The model under review builds one solid part; all positions refer to its coordinate system, in mm. A direction names the side the tool comes from. Coordinates: 2 decimals unless noted, no trailing zeros. Loops run counter-clockwise (first coordinate to the right, second up) from the corner with the lowest first, then second, coordinate; pieces in that order, holes last. Notation, with made-up numbers: M -19,17 L 15,17 A31 ccw 15,56 Z; hole C 35.5,39.5 d5. An arc over 180 degrees is marked long. Write item = value, one per line. Start each with the question number.
Q1. For faces 5 (the face through (12, 7, 3)), 6 (the face through (-7, 8, 2)), 7 (the face through (19, 8, 2)), 8 (the face through (10.566, 5.986, 1.394)), 9 (the face through (11, 7, 1)), list the 3-axis set-ups (+Z, -Z, +X, -X, +Y, -Y) from which the entire face can be reached by the end or side of a thin tool; tool diameter is ignored.
Q2. We need section A-A on y = 7.5. Give the boundary of the cut face in (x, z), and give its area (3 significant figures).
Q3. We need section D-D on y = 13.25. Give the boundary of the cut face in (x, z).
Q4. Wall thickness on probe 1 along Z at (x, y) = (4.5, 3.25); probe 2 along Y at (x, z) = (22, -1.4); probe 3 along X at (y, z) = (3.25, 2.75): over which ranges is each line inside the solid? List them lowest first.
Q5. We need section B-B on z = -1.5. Give the boundary of the cut face in (x, y), and give its area (3 significant figures).
Q6. We need section C-C on x = 26.5. Give the boundary of the cut face in (y, z), and give its area (3 significant figures).
Q7. Clearance check with flat-ended pins moving along their axes: pin 1 Ø3 at (x, z) = (10, 2) entering from -Y; pin 2 Ø3 at (y, z) = (10, 4.5) entering from +X; pin 3 Ø5 at (y, z) = (10.5, 3.5) entering from -X; pin 4 Ø0.8 at (x, z) = (2, 3) entering from +Y. State where each tip first meets the part, or that it passes through.
Q8. Mouldability with a two-part tool opening along X and no side actions: class faces 1 (the face through (11, 5, 1)), 2 (the face through (29.5, 7.66, -0.54)), 3 (the face through (6, 8, -3)), 4 (the face through (6, 7, 0)) as released by +X, released by -X, zero draft, split by the parting line, or undercut.
from build123d import *

# Parameters (mm, degrees)
SKETCH1_W           = 18
SKETCH1_H           = 11
SKETCH1_W_2         = 12
SKETCH1_H_2         = 5
BOSS_EXTRUDE1_DEPTH = 15
SKETCH2_R           = 2.5
BOSS_EXTRUDE2_DEPTH = 5
BOSS_EXTRUDE3_DEPTH = 2


with BuildPart() as part:
    # Sketch1 → Boss-Extrude1 (new body)
    with BuildSketch(Plane(origin=(0, 0, 0), x_dir=(1, 0, 0), z_dir=(0, 1, 0))):
        with Locations((6, -2.5)):
            Rectangle(SKETCH1_W, SKETCH1_H)
        with Locations((6, -2.5)):
            Rectangle(SKETCH1_W_2, SKETCH1_H_2, mode=Mode.SUBTRACT)
    extrude(amount=BOSS_EXTRUDE1_DEPTH)

    # Sketch2 → Boss-Extrude2 (add)
    with BuildSketch(Plane(origin=(0, 0, -3), x_dir=(-1, 0, 0), z_dir=(0, 0, -1))):
        with BuildLine():
            ThreePointArc((10, 15), (17.5, 7.5), (10, 0))
            Line((10, 0), (3, 0))
            Line((3, 0), (3, 15))
            Line((3, 15), (10, 15))
        make_face()
        with Locations((10, 7.5)):
            Circle(SKETCH2_R, mode=Mode.SUBTRACT)
        with BuildLine():
            Line((-15, 15), (-22, 15))
            ThreePointArc((-22, 15), (-29.5, 7.5), (-22, 0))
            Line((-22, 0), (-15, 0))
            Line((-15, 0), (-15, 15))
        make_face()
        with Locations((-22, 7.5)):
            Circle(SKETCH2_R, mode=Mode.SUBTRACT)
    extrude(amount=-BOSS_EXTRUDE2_DEPTH)

    # Sketch3 → Boss-Extrude3 (add)
    with BuildSketch(Plane(origin=(0, 5, 0), x_dir=(-1, 0, 0), z_dir=(0, -1, 0))):
        Polygon((-12, -2.828427125), (-12, 0), (-9.171572875, 0), align=None)
        Polygon((0, -2.171572875), (0, -5), (-2.828427125, -5), align=None)
    extrude(amount=-BOSS_EXTRUDE3_DEPTH)


solid = part.part
Returned:
q1.face_5 = none
q1.face_6 = +Z, -X, +Y, -Y
q1.face_7 = +Z, +X, +Y, -Y
q1.face_8 = +Y, -Y
q1.face_9 = +Y
q2.outline = M -17.5,-3 L -12.5,-3 L -12.5,2 L -17.5,2 Z; M -7.5,-3 L 19.5,-3 L 19.5,2 L 15,2 L 15,8 L -3,8 L -3,2 L -7.5,2 Z; M 24.5,-3 L 29.5,-3 L 29.5,2 L 24.5,2 Z; hole M 0,0 L 12,0 L 12,5 L 0,5 Z
q2.area = 233 mm^2
q3.outline = M -14.82,-3 L 26.82,-3 L 26.82,2 L 15,2 L 15,8 L -3,8 L -3,2 L -14.82,2 Z; hole M 0,0 L 12,0 L 12,5 L 0,5 Z
q4.probe_1 = -3 to 0, 5 to 8
q4.probe_2 = 0 to 5, 10 to 15
q4.probe_3 = -3 to 0, 12 to 15
q5.outline = M -10,0 L 22,0 A7.5 ccw 22,15 L -10,15 A7.5 ccw Z; hole C -10,7.5 d5; hole C 22,7.5 d5
q5.area = 617 mm^2
q6.outline = M 1.5,-3 L 13.5,-3 L 13.5,2 L 1.5,2 Z
q6.area = 60.0 mm^2
q7.pin_1 = 5
q7.pin_2 = 15
q7.pin_3 = -17.43
q7.pin_4 = through
q8.face_1 = undercut
q8.face_2 = released by +X
q8.face_3 = zero draft
q8.face_4 = undercut
